Autodesk Inventor part; units mm, degrees
ref_plane "YZ Plane" through (0, 0, 0) normal (1, 0, 0) x (0, 1, 0)
ref_plane "XZ Plane" through (0, 0, 0) normal (0, 1, 0) x (-1, 0, 0)
ref_plane "XY Plane" through (0, 0, 0) normal (0, 0, 1) x (1, 0, 0)
sketch "Sketch7" plane through (0, 0, 0) normal (0, 1, 0) x (-1, 0, 0)
  line L0 (-204.851, 320.802) -> (-204.851, -320.802)
  line L1 (-204.851, -320.802) -> (49.149, -320.802)
  line L2 (204.851, -165.1) -> (204.851, 165.1)
  line L3 (49.149, 320.802) -> (-204.851, 320.802)
  line L4 (-286.7914, 0) -> (286.7914, 0)
  line L5 (0, -449.1228) -> (0, 449.1228)
  line L6 (172.847, -38.1) -> (-7.493, -38.1)
  line L7 (-7.493, -38.1) -> (-7.493, 38.1)
  line L8 (-7.493, 38.1) -> (172.847, 38.1)
  line L9 (172.847, 38.1) -> (172.847, -38.1)
  circle A0 centre (188.849, 0) radius 3.175
  circle A1 centre (-115.951, 304.8) radius 3.175
  circle A2 centre (-115.951, -304.8) radius 3.175
  line L10 (-27.051, -320.802) -> (-27.051, 320.802) construction
  line L11 (204.851, -70.0665) -> (-27.051, -70.0665) construction
  line L12 (204.851, 0) -> (143.8291, 0) construction
  line L13 (49.149, -320.802) -> (204.851, -165.1)
  line L14 (204.851, 165.1) -> (49.149, 320.802)
  point P0 (0, 0)
  dimension "d22" = 76.2
  dimension "d23" = 180.34
  dimension "d24" = 32.004
  dimension "d25" = 6.35
  dimension "d26" = 16.002
  dimension "d27" = 16.002
  dimension "d28" = 165.1
  dimension "d29" = 641.604
  dimension "d31" = 330.2
  dimension "d32" = 254
  dimension "d36" = 45
  dimension "d37" = 220.1959
  dimension "d38" = 231.902
extrude "Extrusion5" add sketch "Sketch7" along normal blind 5.08 contours L3 L5 L8 L7 L4 L0 | L4 L7 L6 L5 L1 L0 | L3 L14 L2 L4 A0 L9 L8 L5 | L5 L6 L9 L4 A0 L2 L13 L1
equation "\"d28\" = 0.5 * SideLength"
equation "\"d31\" = SideLength"
properties part number "eLECTORNICS bOARD"
Work out the finished part from the listing and answer in its coordinate system (mm). Round coordinates to 2 decimals unless told otherwise and drop trailing zeros. Write each loop counter-clockwise with the first axis right and the second up, starting at its lowest first coordinate (ties: lowest second). Pieces come first, ordered by that corner, then holes.
1) A cutting plane is placed at D-D (z = -202). Give the vertices of the cut face in (x, y), plus the area to 3 significant figures.
2) A cutting plane is placed at B-B (x = -127.5). Give the vertices of the cut face in (y, z), plus the area to 3 significant figures.
3) A cutting plane is placed at C-C (y = 3.8). Give the vertices of the cut face in (x, z) (3 decimals).
4) Given pin 1 Ø1.5 at (y, z) = (2, 192) entering from -X; pin 2 Ø7.5 at (x, z) = (115.951, -304.8) entering from -Y, each flat-ended and moving along its own axis, determine where each tip first touches the part or whether it passes through.
5) Straight lines are drawn through the part: line 1 (X direction, y = 2, z = 0); line 2 (X direction, y = 4.55, z = -19.5); line 3 (Z direction, x = -20.5, y = 3.1). For each, find the intervals that lie inside material, in ascending order.
6) A cutting plane is placed at A-A (z = -19). Give the vertices of the cut face in (x, y).
Completed:
1. outline: (-167.95, 0) - (204.85, 0) - (204.85, 5.08) - (-167.95, 5.08) - close
1. area: 1,890 mm2
2. outline: (0, -242.45) - (5.08, -242.45) - (5.08, -38.1) - (0, -38.1) - close; (0, 38.1) - (5.08, 38.1) - (5.08, 242.45) - (0, 242.45) - close
2. area: 2,080 mm2
3. outline: (-204.851, -165.1) - (-49.149, -320.802) - (204.851, -320.802) - (204.851, 320.802) - (-49.149, 320.802) - (-204.851, 165.1) - close; hole circle Ø6.35 at (-188.849, 0); hole (-172.847, -38.1) - (7.493, -38.1) - (7.493, 38.1) - (-172.847, 38.1) - close; hole circle Ø6.35 at (115.951, -304.8); hole circle Ø6.35 at (115.951, 304.8)
4. pin 1: stops at x = -178.7
4. pin 2: stops at y = 0
5. line 1: x = -204.85 to -192.02, -185.67 to -172.85, 7.49 to 204.85
5. line 2: x = -204.85 to -172.85, 7.49 to 204.85
5. line 3: z = -320.8 to -38.1, 38.1 to 320.8
6. outline: (-204.85, 0) - (-172.85, 0) - (-172.85, 5.08) - (-204.85, 5.08) - close; (7.49, 0) - (204.85, 0) - (204.85, 5.08) - (7.49, 5.08) - close
